Can you work these out from the drawing? Everything is in mm from the part's minimum corner. A direction names the side the tool comes from. Coordinates: 2 decimals unless noted, no trailing zeros. Loops run counter-clockwise (first coordinate to the right, second up) from the corner with the lowest first, then second, coordinate; pieces in that order, holes last. Notation, with made-up numbers: (-3.75, 47.5) - (17.25, 47.5) arc R32 ccw to (17.25, 85.5) - close; hole circle Ø4 at (-5, -8.5). An arc over 180 degrees is marked (long way). Put each result on its own line as item: value. Start each with the question number.
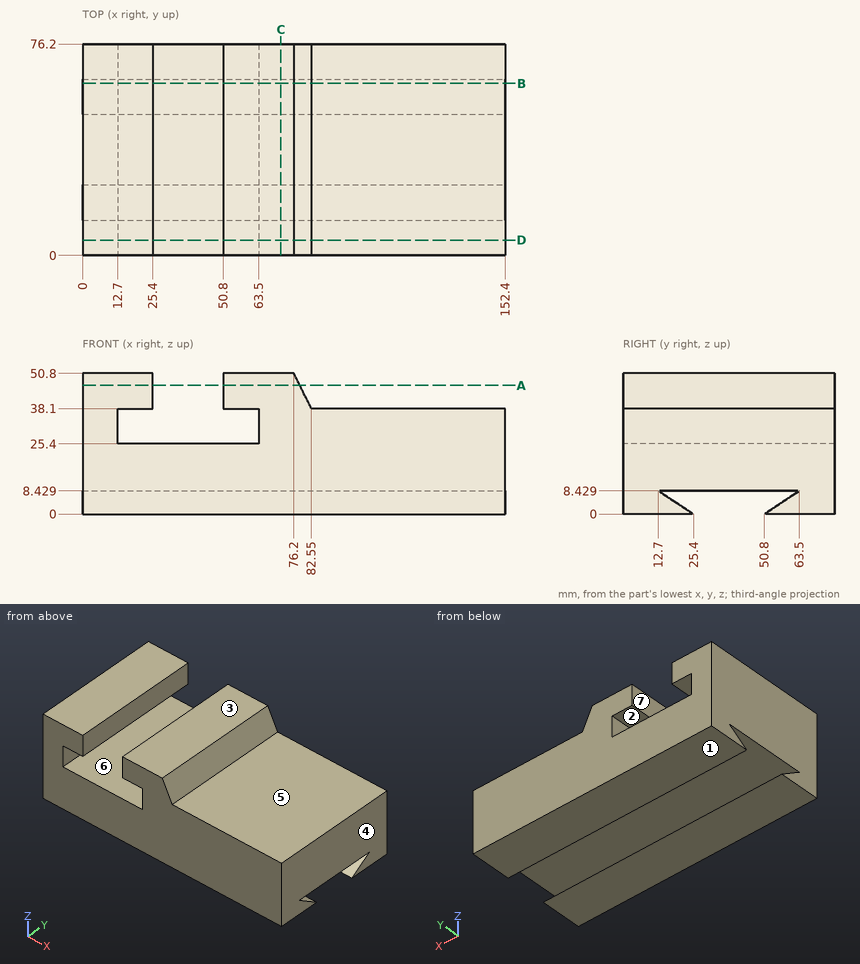
Q1. I want a section at D-D on y = 5.5. List the corners of the cut face in (x, z) for me.
Q2. Please list where these lines run through material, in increasing order: line 1 along X through (y, z) = (13, 32.5); line 2 along Z through (x, y) = (21, 26.5); line 3 along Z through (x, y) = (25, 64.5). Write a range as [from, to].
Q3. Will these pins go through, and if not, where does the flat tip stop? pin 1 (4 mm diameter, centred on y = 51.5, z = 30.5, fed in from -X); pin 2 (14 mm diameter, centred on y = 25.5, z = 47, fed in from +X); pin 3 (6.5 mm diameter, centred on x = 22, y = 40.5, fed in from -Z).
Q4. We'd pull the mould along Z, two halves only. Please class the marked faces 1, 2, 3 and 4: released by +Z, released by -Z, zero draft, split by the parting line, or undercut.
Q5. I want a section at A-A on z = 46.5. List the corners of the cut face in (x, y) for me.
Q6. I want a section at B-B on y = 62. List the corners of the cut face in (x, z) for me.
Q7. On a 3-axis mill with a long thin cutter (end or side, diameter ignored), from which of +Z, -Z, +X, -X, +Y, -Y can I reach the whole of each face in a straight line? I mean the marked faces 5, 6 and 7. Say none if no direction works.
Q8. I want a section at C-C on x = 71.5. List the corners of the cut face in (y, z) for me.
Calculated:
1. outline: (0, 0) - (152.4, 0) - (152.4, 38.1) - (82.55, 38.1) - (76.2, 50.8) - (50.8, 50.8) - (50.8, 38.1) - (63.5, 38.1) - (63.5, 25.4) - (12.7, 25.4) - (12.7, 38.1) - (25.4, 38.1) - (25.4, 50.8) - (0, 50.8) - close
2. line 1: [0, 12.7], [63.5, 152.4]
2. line 2: [8.43, 25.4], [38.1, 50.8]
2. line 3: [0, 25.4], [38.1, 50.8]
3. pin 1: x = 0
3. pin 2: x = 81.6
3. pin 3: z = 8.43
4. face 1: released by -Z
4. face 2: undercut
4. face 3: released by +Z
4. face 4: zero draft
5. outline: (0, 0) - (25.4, 0) - (25.4, 76.2) - (0, 76.2) - close; (50.8, 0) - (78.35, 0) - (78.35, 76.2) - (50.8, 76.2) - close
6. outline: (0, 0) - (152.4, 0) - (152.4, 7.43) - (0, 7.43) - close; (0, 8.43) - (152.4, 8.43) - (152.4, 38.1) - (82.55, 38.1) - (76.2, 50.8) - (50.8, 50.8) - (50.8, 38.1) - (63.5, 38.1) - (63.5, 25.4) - (12.7, 25.4) - (12.7, 38.1) - (25.4, 38.1) - (25.4, 50.8) - (0, 50.8) - close
7. face 5: +Z, +X, +Y, -Y
7. face 6: +Y, -Y
7. face 7: +Z, +Y, -Y
8. outline: (0, 0) - (25.4, 0) - (12.7, 8.43) - (63.5, 8.43) - (50.8, 0) - (76.2, 0) - (76.2, 50.8) - (0, 50.8) - close
